Geometry check sheet. Reference: the model listing, model coordinates, mm. A direction names the side the tool comes from. Round coordinates to 2 decimals unless told otherwise and drop trailing zeros. Order: outer loops, then holes, each group sorted by start corner. A loop starts at its lowest first (then second) coordinate and runs counter-clockwise, first axis right, second up.
(1) Release check for a two-part mould opening along X. For faces 1 (the face through (25.3, 0, 8)), 2 (the face through (42, -20.5, 16)), 3 (the face through (28, -21.5, 8)) record: +X half, -X half, draft (parallel to the pull), parting line (faces both ways), or undercut.
(2) Material ranges on line 1 along X through (y, z) = (3.5, 14); line 2 along Y through (x, z) = (42.5, 13); line 3 along X through (y, z) = (-10, 13.5), recorded low to high.
(3) Set-up check for faces 4 (the face through (49.1, 7, 13)), 5 (the face through (28.6, 0, 7)), 6 (the face through (54, -21.5, 8)), 7 (the face through (31, -21, 8)), 8 (the face through (47, 7, 16)): record each of +Z, -Z, +X, -X, +Y, -Y from which the full face is reachable in a straight line by a thin tool's end or side.
(4) Sectioned sample at B-B (z = 12). Record the boundary of the cut face in (x, y), plus the area to 3 significant figures.
(5) Go/stop test with flat-tipped pins: pin 1 (1.2 mm diameter, centred on x = 39.5, z = 13.5, fed in from -Y); pin 2 (5 mm diameter, centred on x = 35, y = -2.5, fed in from -Z); pin 3 (1.6 mm diameter, centred on x = 40.5, z = 15.5, fed in from -Y). Record where each tip stops, or that it passes through.
(6) Sectioned sample at A-A (y = 15.5). Record the boundary of the cut face in (x, z).
(7) Sectioned sample at D-D (z = 5). Record the boundary of the cut face in (x, y).
(8) Sectioned sample at C-C (x = 36.5). Record the boundary of the cut face in (y, z).
from build123d import *

# Parameters (mm, degrees)
PAD001_DEPTH    = 17
SKETCH008_W     = 25.8
SKETCH008_H     = 41
POCKET005_DEPTH = 15
SKETCH009_W     = 13.3
SKETCH009_H     = 18.7
POCKET006_DEPTH = 5
SKETCH010_W     = 2.3
SKETCH010_H     = 43
PAD002_DEPTH    = 17
SKETCH011_W     = 2
SKETCH011_H     = 18.9
SKETCH011_W_2   = 17.5
SKETCH011_H_2   = 2
PAD003_DEPTH    = 6


with BuildPart() as part:
    # Sketch007 → Pad001 (new body)
    with BuildSketch(Plane.XY):
        Polygon((17.6, 21.5), (45.4, 21.5), (45.4, -21.5), (42, -21.5), (42, -20.5), (21, -20.5), (21, -21.5), (17.6, -21.5), align=None)
    extrude(amount=PAD001_DEPTH)

    # Sketch008 (on Face9 of Pad001) → Pocket005 (cut)
    with BuildSketch(Plane(origin=(0, 0, 0), x_dir=(1, 0, 0), z_dir=(0, 0, -1))):
        with Locations((31.5, 0)):
            Rectangle(SKETCH008_W, SKETCH008_H)
    extrude(amount=-POCKET005_DEPTH, mode=Mode.SUBTRACT)

    # Sketch009 (on Face5 of Pocket005) → Pocket006 (cut)
    with BuildSketch(Plane.XY.offset(17)):
        with Locations((30.35, 7.55)):
            Rectangle(SKETCH009_W, SKETCH009_H)
    extrude(amount=-POCKET006_DEPTH, mode=Mode.SUBTRACT)

    # Sketch010 → Pad002 (join)
    with BuildSketch(Plane.XY):
        with Locations((16.45, 0)):
            Rectangle(SKETCH010_W, SKETCH010_H)
    extrude(amount=PAD002_DEPTH)

    # Sketch011 (on Face5 of Pad002) → Pad003 (join)
    with BuildSketch(Plane.XY.offset(17)):
        with Locations((38.1, 7.55)):
            Rectangle(SKETCH011_W, SKETCH011_H)
        with Locations((22.6, 7.55)):
            Rectangle(SKETCH011_W, SKETCH011_H)
        with Locations((30.35, 18)):
            Rectangle(SKETCH011_W_2, SKETCH011_H_2)
        with Locations((30.35, -2.9)):
            Rectangle(SKETCH011_W_2, SKETCH011_H_2)
    extrude(amount=-PAD003_DEPTH)


with BuildPart() as part_1:
    # Body001 placement: moved
    add(part.part.moved(Location((10, 0, 0))))


solid = part_1.part
Answer below:
1. face 1: -X half
1. face 2: undercut
1. face 3: draft
2. line 1: x = 25.3 to 28.6, 31.6 to 33.6, 47.1 to 49.1, 54.4 to 55.4
2. line 2: y = -3.9 to -1.9, 17 to 19, 20.5 to 21.5
2. line 3: x = 25.3 to 28.6, 54.4 to 55.4
3. face 4: -Z, -Y
3. face 5: -Z
3. face 6: +Z, -Z, +X, -X, -Y
3. face 7: +Z, -Z, -Y
3. face 8: +Z, -Z
4. outline: (25.3, -21.5) - (31, -21.5) - (31, -20.5) - (28.6, -20.5) - (28.6, 20.5) - (54.4, 20.5) - (54.4, -20.5) - (52, -20.5) - (52, -21.5) - (55.4, -21.5) - (55.4, 21.5) - (25.3, 21.5) - close; (31.6, -3.9) - (49.1, -3.9) - (49.1, 19) - (31.6, 19) - close; hole (33.6, -1.9) - (47.1, -1.9) - (47.1, 17) - (33.6, 17) - close
4. area: 361 mm2
5. pin 1: stops at y = -3.9
5. pin 2: stops at z = 11
5. pin 3: stops at y = -20.5
6. outline: (25.3, 0) - (28.6, 0) - (28.6, 15) - (31.6, 15) - (31.6, 11) - (33.6, 11) - (33.6, 15) - (33.7, 15) - (33.7, 17) - (25.3, 17) - close; (47, 15) - (47.1, 15) - (47.1, 11) - (49.1, 11) - (49.1, 15) - (54.4, 15) - (54.4, 0) - (55.4, 0) - (55.4, 17) - (47, 17) - close
7. outline: (25.3, -21.5) - (31, -21.5) - (31, -20.5) - (28.6, -20.5) - (28.6, 20.5) - (54.4, 20.5) - (54.4, -20.5) - (52, -20.5) - (52, -21.5) - (55.4, -21.5) - (55.4, 21.5) - (25.3, 21.5) - close
8. outline: (-20.5, 15) - (-3.9, 15) - (-3.9, 11) - (-1.9, 11) - (-1.9, 15) - (-1.8, 15) - (-1.8, 17) - (-20.5, 17) - close; (16.9, 15) - (17, 15) - (17, 11) - (19, 11) - (19, 15) - (20.5, 15) - (20.5, 0) - (21.5, 0) - (21.5, 17) - (16.9, 17) - close
